Model file for the job. Use its own axes, mm. Face numbers are marked on the shaded views. A direction names the side the tool comes from. Give positions to 0.01 mm unless a question says otherwise; leave off trailing zeros. Order: outer loops, then holes, each group sorted by start corner. A loop starts at its lowest first (then second) coordinate and runs counter-clockwise, first axis right, second up. Notation, with made-up numbers: (72.25, -34.75) - (131.25, -34.75) arc R27 cw to (131.25, -13.75) - close; hole circle Ø9 at (31, 89). An arc over 180 degrees is marked (long way). Return JSON: item names as keys, results as strings. Group by question number.
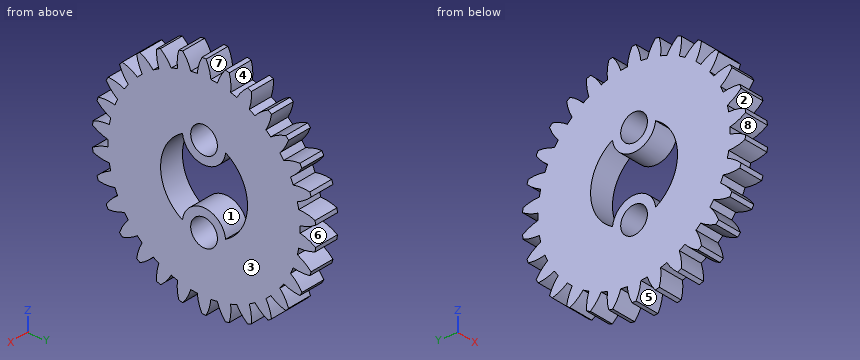
from build123d import *

# Parameters (mm, degrees)
BASPROSKE_W          = 4
BASPROSKE_H          = 18
TOOTHCUT_DEPTH       = 26.768197453
TEETHCUTS_COUNT      = 30
TEETHCUTS_ANGLE      = 348
BORSKE_R             = 7
BORE_DEPTH           = 50.0000508
SKETCH2_R            = 3.5
BOSS_EXTRUDE1_DEPTH  = 4
M4_CLEARANCE_HOLE1_D = 4.3


with BuildPart() as part:
    # BasProSke → Base-Revolve (revolve)
    with BuildSketch(Plane(origin=(0, 0, 0), x_dir=(1, 0, 0), z_dir=(0, 1, 0)), mode=Mode.PRIVATE) as base_revolve_sk:
        with Locations((2, 9)):
            Rectangle(BASPROSKE_W, BASPROSKE_H)
    revolve(base_revolve_sk.sketch.rotate(Axis((-10, 0, 0), (1, 0, 0)), 180), axis=Axis((-10, 0, 0), (1, 0, 0)))

    # TooCutSke → ToothCut (cut, through all)
    with BuildSketch(Plane(origin=(0, 0, 0), x_dir=(0, 0, -1), z_dir=(1, 0, 0))):
        with BuildLine():
            ThreePointArc((0.523521522, 15.458887906), (0, 15.46775), (-0.523521522, 15.458887906))
            ThreePointArc((-0.523521522, 15.458887906), (-0.919551256, 16.760900189), (-1.568701479, 17.957010353))
            ThreePointArc((-1.568701479, 17.957010353), (0, 18.0254), (1.568701479, 17.957010353))
            ThreePointArc((1.568701479, 17.957010353), (0.919551256, 16.760900189), (0.523521522, 15.458887906))
        make_face()
    toothcut = extrude(amount=TOOTHCUT_DEPTH, mode=Mode.SUBTRACT)

    # TeethCuts: ToothCut ×30 about axis
    teethcuts_axis = Axis((-10, 0, 0), (1, 0, 0))
    for i in range(1, TEETHCUTS_COUNT):
        add(toothcut.rotate(teethcuts_axis, i * TEETHCUTS_ANGLE / (TEETHCUTS_COUNT - 1)), mode=Mode.SUBTRACT)

    # BorSke → Bore (cut, symmetric)
    with BuildSketch(Plane(origin=(0, 0, 0), x_dir=(0, 0, -1), z_dir=(1, 0, 0))):
        with Locations(Location((0, 0, 0), (0, 0, 180))):
            Circle(BORSKE_R)
    extrude(amount=BORE_DEPTH, both=True, mode=Mode.SUBTRACT)

    # Sketch2 → Boss-Extrude1 (add)
    with BuildSketch(Plane.ZY):
        with Locations((-6.5, 0)):
            Circle(SKETCH2_R)
        with Locations((6.5, 0)):
            Circle(SKETCH2_R)
    extrude(amount=-BOSS_EXTRUDE1_DEPTH)

    # M4 Clearance Hole1 (through all)
    with Locations(Plane.ZY):
        with Locations((-6.5, 0), (6.5, 0)):
            Hole(M4_CLEARANCE_HOLE1_D / 2)


solid = part.part
(1) Drop flat-ended pins along their axis: pin 1 Ø2 at (x, z) = (1.5, -12.5) entering from +Y; pin 2 Ø1 at (x, z) = (3.5, 1) entering from +Y; pin 3 Ø1.5 at (x, z) = (0.5, 7) entering from -Y. Give the stop position or say it passes through.
(2) 3-axis set-ups, long thin cutter, end or side, ignore diameter. For the marked faces 4, 5, 6, 7 and 8: which of +Z, -Z, +X, -X, +Y, -Y reach the whole face in a straight line?
(3) Pull direction Y, two halves, no side cores. Call the marked faces 1, 2 and 3: released by +Y, released by -Y, zero draft, split by the parting line, or undercut.
(4) Drill centre lines: L1, parallel to Z at x = 3.4, y = -13; L2, parallel to Y at x = 2.1, z = -6.5; L3, parallel to Z at x = 2.8, y = 14.5. Where is each one in solid material? Low to high.
(5) Slice it at B-B (x = 2.2). State how many separate pieces and enclosed holes the cut face has, and give its area (3 significant figures).
(6) Slice it at A-A (y = -6.5). Give the cut face in (x, z).
Result set:
{
 "1": {"pin 1": "stops at y = 13.6", "pin 2": "stops at y = 17.85", "pin 3": "stops at y = -15.02"},
 "2": {"face 4": "+X, -X", "face 5": "-Z, +X, -X", "face 6": "+X, -X, +Y", "face 7": "+Z, +X, -X", "face 8": "+X, -X, -Y"},
 "3": {"face 1": "undercut", "face 2": "released by -Y", "face 3": "zero draft"},
 "4": {"L1": "z = -12.25 to -10.56, -8.75 to 8.75, 10.56 to 12.25", "L2": "y = -14.04 to -2.15, 2.15 to 14.04", "L3": "z = -9.19 to -7.23, -5.84 to 5.84, 7.23 to 9.19"},
 "5": {"separate pieces": "1", "enclosed holes": "3", "area": "733 mm²"},
 "6": {"outline": "(0, -16.13) - (4, -16.13) - (4, -2.6) - (0, -2.6) - close; (0, 2.6) - (4, 2.6) - (4, 16.13) - (0, 16.13) - close"}
}
